Autodesk Inventor part; units mm, degrees
ref_plane "YZ Plane" through (0, 0, 0) normal (1, 0, 0) x (0, 1, 0)
ref_plane "XZ Plane" through (0, 0, 0) normal (0, 1, 0) x (-1, 0, 0)
ref_plane "XY Plane" through (0, 0, 0) normal (0, 0, 1) x (1, 0, 0)
sketch "Boceto1" plane through (0, 0, 0) normal (0, 0, 1) x (1, 0, 0)
  line L0 (0, -83.5) -> (0, 83.5)
  line L1 (0, 83.5) -> (-1.5, 83.5)
  line L2 (-1.5, 83.5) -> (-1.5, 74.5)
  line L3 (-1.5, 74.5) -> (-3, 74.5)
  line L4 (-3, 74.5) -> (-3, -48.5)
  line L5 (-3, -48.5) -> (-1.5, -48.5)
  line L6 (-1.5, -48.5) -> (-1.5, -83.5)
  line L7 (-1.5, -83.5) -> (0, -83.5)
  point P0 (0, 0)
  point P1 (0, 0)
  dimension "d1" = 3
  dimension "d2" = 6
  dimension "d3" = 9
  dimension "d4" = 123
  dimension "d8" = 35
revolve "Revolución1" add sketch "Boceto1" angle 360 about axis through (0, -83.5, 0) along (0, 1, 0)
thread "Rosca1"
chamfer "Chaflán1" distance 0.3067 angle 45 2 edges at (1.5, 83.5, 0) (1.5, -83.5, 0)
properties part number "Columnas" material "Aluminio 6061"
Could you check a few things on this model? Use its own coordinates, in mm. A direction names the side the tool comes from. Coordinates: 2 decimals unless noted, no trailing zeros. Order: outer loops, then holes, each group sorted by start corner. A loop starts at its lowest first (then second) coordinate and runs counter-clockwise, first axis right, second up. Notation, with made-up numbers: M -28,-36 L -5,-36 A12 ccw -5,-31 Z; hole C -1,-22 d4. An arc over 180 degrees is marked long. Use a Markdown table: item, result. Add a question column.
Q1. I want a section at D-D on y = 60.5. List the corners of the cut face in (x, z) for me.
Q2. If I drill on L1, parallel to Y at x = 1.45, z = -0.55; L2, parallel to Z at x = 2.6, y = -28.5; L3, parallel to X at y = 74, z = 0.2, over which ranges is the centre line in solid material (lowest first)?
Q3. I want a section at C-C on y = -56. List the corners of the cut face in (x, z) for me.
Q4. I'm going to push a flat-ended pin straight in: pin 1 (3 mm diameter, centred on y = -56.5, z = 0.5, fed in from +X). Where does the tip first touch, or does it pass through?
Q5. I want a section at B-B on z = 0. List the corners of the cut face in (x, y) for me.
Q6. I want a section at A-A on x = 0. List the corners of the cut face in (y, z) for me.
Q7. Which directions (+Z, -Z, +X, -X, +Y, -Y) give clear straight access to the entire face, cutting with the end or side of a thin tool? Please do faces 1 (the cylindrical face through (3, 12, 0)), 2 (the flat face through (-1.3, 74.5, -1.3)), 3 (the flat face through (-1.3, -48.5, -1.3)).
Checked values:
| question | item | result |
|---|---|---|
| 1 | outline | C 0,0 d6 |
| 2 | L1 | -48.5 to 74.5 |
| 2 | L2 | -1.5 to 1.5 |
| 2 | L3 | -2.99 to 2.99 |
| 3 | outline | C 0,0 d3 |
| 4 | pin 1 | x = 1.5 |
| 5 | outline | M -3,-48.5 L -1.5,-48.5 L -1.5,-83.19 L -1.19,-83.5 L 1.19,-83.5 L 1.5,-83.19 L 1.5,-48.5 L 3,-48.5 L 3,74.5 L 1.5,74.5 L 1.5,83.19 L 1.19,83.5 L -1.19,83.5 L -1.5,83.19 L -1.5,74.5 L -3,74.5 Z |
| 6 | outline | M -83.5,-1.19 L -83.19,-1.5 L -48.5,-1.5 L -48.5,-3 L 74.5,-3 L 74.5,-1.5 L 83.19,-1.5 L 83.5,-1.19 L 83.5,1.19 L 83.19,1.5 L 74.5,1.5 L 74.5,3 L -48.5,3 L -48.5,1.5 L -83.19,1.5 L -83.5,1.19 Z |
| 7 | face 1 | +Y, -Y |
| 7 | face 2 | +Y |
| 7 | face 3 | -Y |
